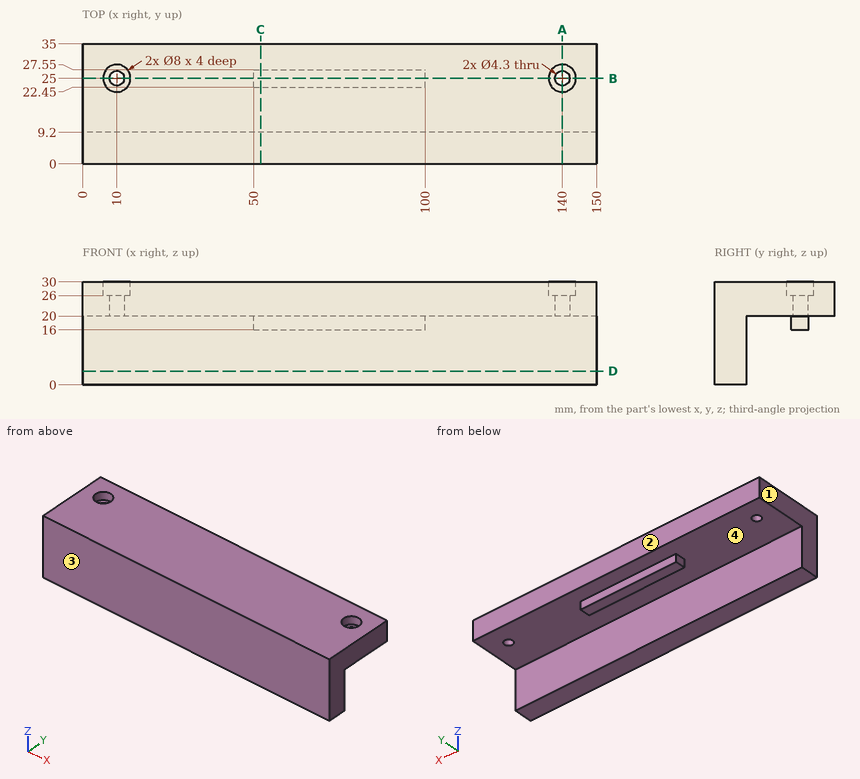
Geometry: see drawing. Coordinates: mm, zero at the bounding-box minimum. Coordinates: 2 decimals unless noted, no trailing zeros. Write each loop counter-clockwise with the first axis right and the second up, starting at its lowest first coordinate (ties: lowest second). Pieces come first, ordered by that corner, then holes.
1) Section B-B on y = 25. Output: boundary loops of the cut face in (x, z), and give its area (3 significant figures).
2) Section D-D on z = 4. Output: boundary loops of the cut face in (x, y).
3) Section A-A on x = 140. Output: boundary loops of the cut face in (y, z), and give its area (3 significant figures).
4) Mould query, pull axis Y, two halves, no side actions, for the marked faces 1, 2, 3 and 4. Classes: pulls with the +Y half, pulls with the -Y half, needs draft (parallel to the pull), parting line crosses it, or undercut.
5) Pin query (flat end, axial travel): pin 1 Ø16 at (x, z) = (94, 10.5) entering from +Y; pin 2 Ø5.5 at (x, y) = (83, 24.5) entering from -Z; pin 3 Ø4 at (x, y) = (141.5, 24.5) entering from +Z; pin 4 Ø3 at (y, z) = (30.5, 16.5) entering from +X. Return the tip coordinate at first contact, or that it passes through.
6) Section C-C on x = 52. Output: boundary loops of the cut face in (y, z), and give its area (3 significant figures).
7) Material intervals for line 1 along Z through (x, y) = (143.5, 26); line 2 along Z through (x, y) = (16.5, 9.5); line 3 along Y through (x, z) = (10, 23.35), sorted ascending.
Check result:
1. outline: (0, 20) - (7.85, 20) - (7.85, 26) - (6, 26) - (6, 30) - (0, 30) - close; (12.15, 20) - (50, 20) - (50, 16) - (100, 16) - (100, 20) - (137.85, 20) - (137.85, 26) - (136, 26) - (136, 30) - (14, 30) - (14, 26) - (12.15, 26) - close; (142.15, 20) - (150, 20) - (150, 30) - (144, 30) - (144, 26) - (142.15, 26) - close
1. area: 1,580 mm2
2. outline: (0, 0) - (150, 0) - (150, 9.2) - (0, 9.2) - close
3. outline: (0, 0) - (9.2, 0) - (9.2, 20) - (22.85, 20) - (22.85, 26) - (21, 26) - (21, 30) - (0, 30) - close; (27.15, 20) - (35, 20) - (35, 30) - (29, 30) - (29, 26) - (27.15, 26) - close
3. area: 476 mm2
4. face 1: needs draft
4. face 2: pulls with the +Y half
4. face 3: pulls with the -Y half
4. face 4: undercut
5. pin 1: stops at y = 27.55
5. pin 2: stops at z = 16
5. pin 3: stops at z = 26
5. pin 4: passes through
6. outline: (0, 0) - (9.2, 0) - (9.2, 20) - (22.45, 20) - (22.45, 16) - (27.55, 16) - (27.55, 20) - (35, 20) - (35, 30) - (0, 30) - close
6. area: 554 mm2
7. line 1: z = 20 to 26
7. line 2: z = 20 to 30
7. line 3: y = 0 to 22.85, 27.15 to 35
